For this review, take the finished solid that the model builds, in its own axes (mm). Coordinates: 2 decimals unless noted, no trailing zeros. Loops run counter-clockwise (first coordinate to the right, second up) from the corner with the lowest first, then second, coordinate; pieces in that order, holes last. Notation, with made-up numbers: (56, 40.25) - (114, 40.25) arc R31 ccw to (114, 65.25) - close; hole circle Ø8 at (13, 40). An arc over 180 degrees is marked (long way). Use one line per item in the form item = value. Start each with the question number.
1. Draft analysis for pull direction X (two halves, no side actions). For faces 1 (the face through (125, 0, 6)), 2 (the face through (0, 138, 6)), 3 (the face through (254, 138, 6)), 4 (the face through (182.343, 26.831, 6.261)), state which applies: +X half, -X half, draft (parallel to the pull), parting line (faces both ways), or undercut.
2. Add section A-A on x = 76.2. Give the boundary of the cut face in (y, z), and give its area (3 significant figures).
3. To check wall thickness, follow probe 1 along X at (y, z) = (40.9, 7.75); probe 2 along X at (y, z) = (127, 5); probe 3 along X at (y, z) = (25, 3). State the ranges of each line that lie inside material, in increasing order.
```python
from build123d import *

# Parameters (mm, degrees)
SKETCH1_W           = 254
SKETCH1_H           = 279.4
SKETCH1_R           = 1.5875
SKETCH1_R_2         = 4.7625
SKETCH1_R_3         = 11
BOSS_EXTRUDE1_DEPTH = 12.7


with BuildPart() as part:
    # Sketch1 → Boss-Extrude1 (new body)
    with BuildSketch(Plane.XY):
        with Locations((127, 139.7)):
            Rectangle(SKETCH1_W, SKETCH1_H)
        with Locations((6.35, 25.4)):
            Circle(SKETCH1_R, mode=Mode.SUBTRACT)
        with Locations((247.65, 25.4)):
            Circle(SKETCH1_R, mode=Mode.SUBTRACT)
        with Locations((6.35, 76.2)):
            Circle(SKETCH1_R, mode=Mode.SUBTRACT)
        with Locations((247.65, 76.2)):
            Circle(SKETCH1_R, mode=Mode.SUBTRACT)
        with Locations((6.35, 127)):
            Circle(SKETCH1_R, mode=Mode.SUBTRACT)
        with Locations((247.65, 127)):
            Circle(SKETCH1_R, mode=Mode.SUBTRACT)
        with Locations((6.35, 177.8)):
            Circle(SKETCH1_R, mode=Mode.SUBTRACT)
        with Locations((247.65, 177.8)):
            Circle(SKETCH1_R, mode=Mode.SUBTRACT)
        with Locations((76.2, 25.4)):
            Circle(SKETCH1_R_2, mode=Mode.SUBTRACT)
        with Locations((177.8, 25.4)):
            Circle(SKETCH1_R_2, mode=Mode.SUBTRACT)
        with Locations((127, 25.4)):
            Circle(SKETCH1_R_3, mode=Mode.SUBTRACT)
        with Locations((142.499999988, 40.899999988)):
            Circle(SKETCH1_R, mode=Mode.SUBTRACT)
        with Locations((111.511999988, 40.899999988)):
            Circle(SKETCH1_R, mode=Mode.SUBTRACT)
        with Locations((142.499999988, 9.911999988)):
            Circle(SKETCH1_R, mode=Mode.SUBTRACT)
        with Locations((111.511999988, 9.911999988)):
            Circle(SKETCH1_R, mode=Mode.SUBTRACT)
        with Locations((6.35, 228.6)):
            Circle(SKETCH1_R, mode=Mode.SUBTRACT)
        with Locations((247.65, 228.6)):
            Circle(SKETCH1_R, mode=Mode.SUBTRACT)
        with Locations((6.35, 267.208)):
            Circle(SKETCH1_R, mode=Mode.SUBTRACT)
        with Locations((247.65, 267.208)):
            Circle(SKETCH1_R, mode=Mode.SUBTRACT)
    extrude(amount=BOSS_EXTRUDE1_DEPTH)


solid = part.part
```
Conclusion:
q1.face_1 = draft
q1.face_2 = -X half
q1.face_3 = +X half
q1.face_4 = undercut
q2.outline = (0, 0) - (20.64, 0) - (20.64, 12.7) - (0, 12.7) - close; (30.16, 0) - (279.4, 0) - (279.4, 12.7) - (30.16, 12.7) - close
q2.area = 3,430 mm^2
q3.probe_1 = 0 to 109.92, 113.1 to 140.91, 144.09 to 254
q3.probe_2 = 0 to 4.76, 7.94 to 246.06, 249.24 to 254
q3.probe_3 = 0 to 4.81, 7.89 to 71.45, 80.95 to 116.01, 137.99 to 173.05, 182.55 to 246.11, 249.19 to 254
